Could you check a few things on this model? Use its own coordinates, in mm. Face numbers are marked on the shaded views. A direction names the side the tool comes from. Round coordinates to 2 decimals unless told otherwise and drop trailing zeros. Write each loop counter-clockwise with the first axis right and the second up, starting at its lowest first coordinate (ties: lowest second). Pieces come first, ordered by that corner, then holes. Notation, with made-up numbers: (9.25, -2.5) - (18.25, -2.5) arc R21 cw to (18.25, 1.5) - close; hole circle Ø2 at (-13, 78.25). An arc over 180 degrees is marked (long way). Write each question's results on one line, items separated by ' | '. Start each with the question number.
(1) For P1, Ø8, axis at x = 26, y = 10.5, coming from the +Z side (3 decimals); P2, Ø6, axis at x = 24, z = 9.5, coming from the +Y side; P3, Ø3, axis at x = 21.5, z = 24, coming from the +Y side (3 decimals), each with a flat end and sliding along its axis, tell me the tip position at first contact or that it passes through.
(2) Imagine slicing it at B-B on x = 5. Write out the boundary of the cut face in (y, z) (3 decimals).
(3) On a 3-axis mill with a long thin cutter (end or side, diameter ignored), from which of +Z, -Z, +X, -X, +Y, -Y can I reach the whole of each face in a straight line? I mean the marked faces 4, 5, 6 and 7. Say none if no direction works.
(4) Imagine slicing it at A-A on y = 27.5. Write out the boundary of the cut face in (x, z) (3 decimals).
(5) Please list where these lines run through material, in increasing order: line 1 (Z direction, x = 11, y = 36.5) (3 decimals); line 2 (X direction, y = -8.5, z = -4) (3 decimals); line 3 (Z direction, x = 2, y = 11) (3 decimals). Write a range as [from, to].
(6) Thinking about a two-plate mould opening in X: for the marked faces 1, 2 and 3, which applies, +X half, -X half, draft (parallel to the pull), parting line (faces both ways), or undercut?
(7) Imagine slicing it at C-C on z = 25. Write out the boundary of the cut face in (x, y) (3 decimals), then the cut area to 3 significant figures.
(8) Imagine slicing it at D-D on x = 16. Write out the boundary of the cut face in (y, z) (3 decimals), then the cut area to 3 significant figures.
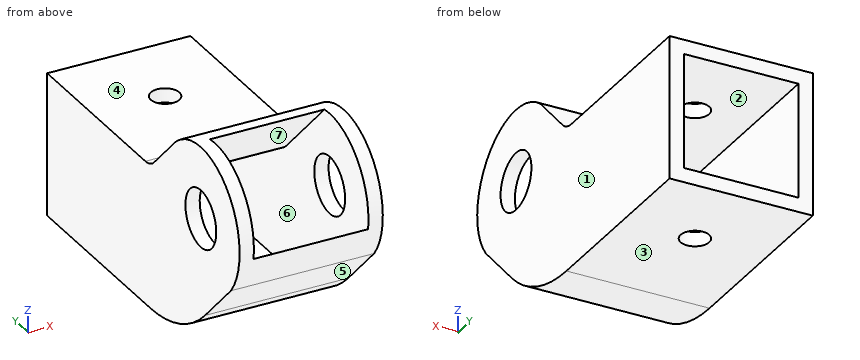
```python
from build123d import *

# Parameters (mm, degrees)
BOSS_EXTRUDE1_DEPTH = 31.75
CUT_EXTRUDE2_START  = -3.175
CUT_EXTRUDE2_DEPTH  = 25.4
SKETCH4_W           = 25.4
SKETCH4_H           = 25.4
CUT_EXTRUDE3_DEPTH  = 3.175
SKETCH6_W           = 25.4
SKETCH6_H           = 25.4
CUT_EXTRUDE5_DEPTH  = 3.175
FILLET1_R           = 5
CUT_EXTRUDE6_REACH  = 79.895
SKETCH8_R           = 3.175
CUT_EXTRUDE7_REACH  = 69.69
SKETCH9_R           = 6.35
CUT_EXTRUDE8_DEPTH  = 68.689586975


with BuildPart() as part:
    # Sketch1 → Boss-Extrude1 (new body)
    with BuildSketch(Plane(origin=(0, 0, 0), x_dir=(0, 0, -1), z_dir=(1, 0, 0))):
        with BuildLine():
            Line((15.875, 42.5), (-15.875, 42.5))
            Line((-15.875, 42.5), (-15.875, 0))
            Line((-15.875, 0), (-38.855970389, -22.980970389))
            Line((-38.855970389, -22.980970389), (-16.405330086, -45.431610691))
            Line((-16.405330086, -45.431610691), (6.575640303, -22.450640303))
            ThreePointArc((6.575640303, -22.450640303), (13.458175157, -12.150198978), (15.875, 0))
            Line((15.875, 0), (15.875, 42.5))
        make_face()
    extrude(amount=BOSS_EXTRUDE1_DEPTH)

    # Sketch3 → Cut-Extrude2 (cut)
    with BuildSketch(Plane.ZY.offset(CUT_EXTRUDE2_START)):
        with BuildLine():
            Line((16.405330086, -40.941482631), (34.365842328, -22.980970389))
            Line((34.365842328, -22.980970389), (12.7, -1.315128061))
            Line((12.7, -1.315128061), (12.7, 39.325))
            Line((12.7, 39.325), (-12.7, 39.325))
            Line((-12.7, 39.325), (-12.7, 0))
            ThreePointArc((-12.7, 0), (-10.524857642, -10.93517908), (-4.330576272, -20.205576272))
            Line((-4.330576272, -20.205576272), (16.405330086, -40.941482631))
        make_face()
    extrude(amount=-CUT_EXTRUDE2_DEPTH, mode=Mode.SUBTRACT)

    # Sketch4 → Cut-Extrude3 (cut)
    with BuildSketch(Plane(origin=(0, 42.5, 0), x_dir=(1, 0, 0), z_dir=(0, 1, 0))):
        with Locations((15.875, 0)):
            Rectangle(SKETCH4_W, SKETCH4_H)
    extrude(amount=-CUT_EXTRUDE3_DEPTH, mode=Mode.SUBTRACT)

    # Sketch6 → Cut-Extrude5 (cut)
    with BuildSketch(Plane(origin=(0, -30.918470389, 30.918470389), x_dir=(1, 0, 0), z_dir=(0, -0.7071067811865518, 0.7071067811865434))):
        with Locations((15.875, -4.649679849)):
            Rectangle(SKETCH6_W, SKETCH6_H)
    extrude(amount=-CUT_EXTRUDE5_DEPTH, mode=Mode.SUBTRACT)

    # Fillet1
    fillet1_edges = [part.edges().sort_by_distance(p)[0] for p in [
        (15.875, 0, 15.875),
        (15.875, -1.315128061, 12.7),
    ]]
    fillet(fillet1_edges, radius=FILLET1_R)

    # Cut-Extrude6: up to this face of the body (flat: up to its plane)
    cut_extrude6_end = Plane(part.part.faces().sort_by_distance((15.875, 22.285533906, 15.875))[0])
    # Sketch8 → Cut-Extrude6 (cut, up to the picked face)
    with BuildSketch(Plane(origin=(0, 0, -15.875), x_dir=(-1, 0, 0), z_dir=(0, 0, -1)), mode=Mode.PRIVATE) as cut_extrude6_sk1:
        with Locations((-15.875, 23.45)):
            Circle(SKETCH8_R)
    cut_extrude6_tool1 = split(extrude(cut_extrude6_sk1.sketch, amount=-CUT_EXTRUDE6_REACH, mode=Mode.PRIVATE), bisect_by=cut_extrude6_end, keep=Keep.BOTH, mode=Mode.PRIVATE)
    add(cut_extrude6_tool1.solids().sort_by(Axis((15.875, 23.45, -15.875), (0, 0, 1)))[0], mode=Mode.SUBTRACT)

    # Cut-Extrude7: up to this face of the body (flat: up to its plane)
    cut_extrude7_end = Plane(part.part.faces().sort_by_distance((0, 0.759502888, 5.54562078))[0])
    # Sketch9 → Cut-Extrude7 (cut, up to the picked face)
    with BuildSketch(Plane(origin=(31.75, 0, 0), x_dir=(0, 0, -1), z_dir=(1, 0, 0)), mode=Mode.PRIVATE) as cut_extrude7_sk1:
        with Locations(Location((-14.160266056, -20.735906358, 0), (0, 0, 180))):
            Circle(SKETCH9_R)
    cut_extrude7_tool1 = split(extrude(cut_extrude7_sk1.sketch, amount=-CUT_EXTRUDE7_REACH, mode=Mode.PRIVATE), bisect_by=cut_extrude7_end, keep=Keep.BOTH, mode=Mode.PRIVATE)
    add(cut_extrude7_tool1.solids().sort_by(Axis((31.75, -20.735906, 14.160266), (-1, 0, 0)))[0], mode=Mode.SUBTRACT)

    # Sketch11 → Cut-Extrude8 (cut, through all)
    with BuildSketch(Plane(origin=(31.75, 0, 0), x_dir=(0, 0, -1), z_dir=(1, 0, 0))):
        with BuildLine():
            ThreePointArc((-4.10994949, -33.136230095), (-25.446915068, -32.022555371), (-26.560589793, -10.685589793))
            Line((-26.560589793, -10.685589793), (-38.855970389, -22.980970389))
            Line((-38.855970389, -22.980970389), (-16.405330086, -45.431610691))
            Line((-16.405330086, -45.431610691), (-4.10994949, -33.136230095))
        make_face()
    extrude(amount=-CUT_EXTRUDE8_DEPTH, mode=Mode.SUBTRACT)


solid = part.part
```
Response:
1) P1: z = 15.875 | P2: y = -31.04 | P3: y = -6.625
2) outline: (-36.553, 12.017) arc R15.962 ccw to (-33.136, 4.11) - (-22.451, -6.576) arc R31.75 ccw to (0, -15.875) - (42.5, -15.875) - (42.5, -12.7) - (0, -12.7) arc R28.575 cw to (-20.206, -4.331) - close; (-18.593, 29.977) - (-2.78, 14.164) arc R5 ccw to (0.756, 12.7) - (42.5, 12.7) - (42.5, 15.875) - (2.071, 15.875) arc R5 cw to (-1.464, 17.339) - (-10.686, 26.561) arc R15.962 ccw to start
3) face 4: +Z, +X, -X, +Y | face 5: -Z, +X, -X, -Y | face 6: none | face 7: -Y
4) outline: (0, -15.875) - (31.75, -15.875) - (31.75, 15.875) - (0, 15.875) - close; hole (3.175, -12.7) - (28.575, -12.7) - (28.575, 12.7) - (3.175, 12.7) - close
5) line 1: [-15.875, -12.7], [12.7, 15.875] | line 2: [0, 3.175], [28.575, 31.75] | line 3: [-15.875, 15.875]
6) face 1: +X half | face 2: undercut | face 3: draft
7) outline: (0, -32.452) - (3.175, -32.452) - (3.175, -13.615) - (28.575, -13.615) - (28.575, -32.452) - (31.75, -32.452) - (31.75, -9.125) - (0, -9.125) - close | area: 262 mm²
8) outline: (-36.553, 12.017) arc R15.962 ccw to (-33.136, 4.11) - (-22.451, -6.576) arc R31.75 ccw to (0, -15.875) - (20.277, -15.875) - (20.277, -12.7) - (0, -12.7) arc R28.575 cw to (-20.206, -4.331) - close; (-18.593, 29.977) - (-2.78, 14.164) arc R5 ccw to (0.756, 12.7) - (20.277, 12.7) - (20.277, 15.875) - (2.071, 15.875) arc R5 cw to (-1.464, 17.339) - (-10.686, 26.561) arc R15.962 ccw to start; (26.623, -15.875) - (42.5, -15.875) - (42.5, -12.7) - (26.623, -12.7) - close; (26.623, 12.7) - (42.5, 12.7) - (42.5, 15.875) - (26.623, 15.875) - close | area: 437 mm²
